Read the model definition and answer for the solid it produces. Units are mm, in the model's axes. Face numbers are marked on the shaded views. A direction names the side the tool comes from. Round coordinates to 2 decimals unless told otherwise and drop trailing zeros. Order: outer loops, then holes, each group sorted by start corner. A loop starts at its lowest first (then second) coordinate and runs counter-clockwise, first axis right, second up. Notation, with made-up numbers: (63.25, 65) - (69.25, 65) arc R16 ccw to (69.25, 93) - close; hole circle Ø7 at (21.25, 5.25). An arc over 180 degrees is marked (long way). One line per question, with ' | ' between items. Start each with the question number.
1) The part is cut by section A-A, the plane z = -6. Give the vertices of the cut face in (x, y), plus the area to 3 significant figures.
2) The mould has two halves that part along X. Classify the marked faces 6, 7, 8 and 9: pulls with the +X half, pulls with the -X half, needs draft (parallel to the pull), parting line crosses it, or undercut.
3) The part is cut by section B-B, the plane x = 31.1. Give the vertices of the cut face in (y, z).
4) The part is cut by section D-D, the plane y = -16.25. Give the vertices of the cut face in (x, z).
5) For the marked faces 1, 2, 3, 4 and 5, determine the directions among +Z, -Z, +X, -X, +Y, -Y from which every point of the face is accessible in a straight line to the end or side of a thin tool.
6) The part is cut by section C-C, the plane z = -10.5. Give the vertices of the cut face in (x, y).
7) Flat-ended cylindrical pins translate along their axes: pin 1 (3 mm diameter, centred on x = 31.1, y = -8.65, fed in from -Z); pin 2 (5 mm diameter, centred on x = 21, z = -32.5, fed in from +Y); pin 3 (4 mm diameter, centred on x = 31.5, z = -9, fed in from -Y); pin 4 (2.5 mm diameter, centred on x = 9.1, y = -8.65, fed in from -Z). Find the tip coordinate at first contact, or state that the pin passes through.
8) Straight lines are drawn through the part: line 1 (Z direction, x = 2, y = -14.25); line 2 (Z direction, x = 16, y = -10); line 3 (X direction, y = -3.35, z = -36.05). For each, find the intervals that lie inside material, in ascending order. Write a range as from..to.
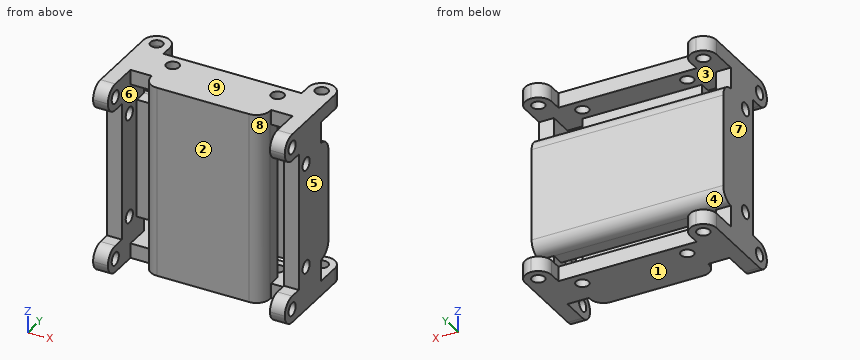
from build123d import *

# Parameters (mm, degrees)
ESBO_O1_R                  = 1.35
RESSALTO_EXTRUS_O1_DEPTH   = 2
ESBO_O3_W                  = 40.2
ESBO_O3_H                  = 2
RESSALTO_EXTRUS_O2_DEPTH   = 10.08
ESBO_O4_W                  = 3.1
ESBO_O4_H                  = 12.84
RESSALTO_EXTRUS_O3_DEPTH   = 34
CORTE_EXTRUS_O1_DEPTH      = 55.735280213
CORTE_EXTRUS_O1_DEPTH_BACK = 55.735280213
ESBO_O5_R                  = 1.35
ESBO_O7_W                  = 37.1
ESBO_O7_H                  = 3.24
CORTE_EXTRUS_O2_DEPTH      = 2
RESSALTO_EXTRUS_O5_START   = 2
ESBO_O12_R                 = 1.35
RESSALTO_EXTRUS_O5_DEPTH   = 2
ESBO_O18_W                 = 3.1
ESBO_O18_H                 = 3.24
RESSALTO_EXTRUS_O6_DEPTH   = 2
ESBO_O19_W                 = 3.1
ESBO_O19_H                 = 3.24
RESSALTO_EXTRUS_O7_DEPTH   = 2
ESBO_O21_R                 = 1.301764144
ESBO_O21_R_2               = 1.35
RESSALTO_EXTRUS_O8_DEPTH   = 1.1
RESSALTO_EXTRUS_O9_START   = 1.1
ESBO_O22_R                 = 1.35
RESSALTO_EXTRUS_O9_DEPTH   = 1.1
ESBO_O23_W                 = 3.1
ESBO_O23_H                 = 5.6
RESSALTO_EXTRUS_O10_DEPTH  = 5.85
CORTE_EXTRUS_O3_REACH      = 63.173
ESBO_O24_R                 = 1.35
ESBO_O25_W                 = 4.5
ESBO_O25_H                 = 3.1
CORTE_EXTRUS_O6_DEPTH      = 4.48
ESBO_O27_W                 = 3.1
ESBO_O27_H                 = 29
CORTE_EXTRUS_O7_DEPTH      = 4.48
ESBO_O28_W                 = 25
ESBO_O28_H                 = 40.2
CORTE_EXTRUS_O8_DEPTH      = 1.24
ESBO_O29_W                 = 25
ESBO_O29_H                 = 5.6
RESSALTO_EXTRUS_O11_DEPTH  = 34
ESBO_O31_W                 = 3.1
ESBO_O31_H                 = 25
RESSALTO_EXTRUS_O12_DEPTH  = 2.84
ESBO_O32_W                 = 25
ESBO_O32_H                 = 5.6
RESSALTO_EXTRUS_O13_DEPTH  = 34
FILETE1_R                  = 2.84
ESBO_O33_W                 = 5.6
ESBO_O33_H                 = 3.1
CORTE_EXTRUS_O9_DEPTH      = 0.55
ESBO_O35_W                 = 3.1
ESBO_O35_H                 = 5.6
CORTE_EXTRUS_O10_DEPTH     = 5.03
FILETE2_R                  = 2.8


with BuildPart() as part:
    # Esboço1 → Ressalto-extrusão1 (new body)
    with BuildSketch(Plane.XY):
        Polygon((0, 0), (5.6, 0), (5.6, -5.85), (34.6, -5.85), (34.6, 0), (40.2, 0), (40.2, -11.45), (0, -11.45), align=None)
        with Locations((2.8, -3.35)):
            Circle(ESBO_O1_R, mode=Mode.SUBTRACT)
        with Locations((37.4, -3.35)):
            Circle(ESBO_O1_R, mode=Mode.SUBTRACT)
        with Locations((31.1, -8.65)):
            Circle(ESBO_O1_R, mode=Mode.SUBTRACT)
        with Locations((9.1, -8.65)):
            Circle(ESBO_O1_R, mode=Mode.SUBTRACT)
    extrude(amount=RESSALTO_EXTRUS_O1_DEPTH)

    # Esboço3 → Ressalto-extrusão2 (add)
    with BuildSketch(Plane.XZ.offset(11.45)):
        with Locations((20.1, 1)):
            Rectangle(ESBO_O3_W, ESBO_O3_H)
    extrude(amount=RESSALTO_EXTRUS_O2_DEPTH)

    # Esboço4 → Ressalto-extrusão3 (add)
    with BuildSketch(Plane(origin=(0, 0, 0), x_dir=(-1, 0, 0), z_dir=(0, 0, -1))):
        with Locations((-38.65, -15.11)):
            Rectangle(ESBO_O4_W, ESBO_O4_H)
        with Locations((-1.55, -15.11)):
            Rectangle(ESBO_O4_W, ESBO_O4_H)
    extrude(amount=RESSALTO_EXTRUS_O3_DEPTH)

    # Esboço5 → Corte-extrusão1 (cut, two sides: drawn at the far end of the back side and taken through both)
    with BuildSketch(Plane.ZY.offset(-37.1).offset(-CORTE_EXTRUS_O1_DEPTH_BACK)):
        with Locations((-6, -14.25)):
            Circle(ESBO_O5_R)
        with Locations((-28, -14.25)):
            Circle(ESBO_O5_R)
    extrude(amount=CORTE_EXTRUS_O1_DEPTH + CORTE_EXTRUS_O1_DEPTH_BACK, mode=Mode.SUBTRACT)

    # Esboço7 → Corte-extrusão2 (cut)
    with BuildSketch(Plane(origin=(0, 0, 0), x_dir=(-1, 0, 0), z_dir=(0, 0, -1))):
        with Locations((-18.55, -19.91)):
            Rectangle(ESBO_O7_W, ESBO_O7_H)
    extrude(amount=-CORTE_EXTRUS_O2_DEPTH, mode=Mode.SUBTRACT)

    # Esboço12 → Ressalto-extrusão5 (add)
    with BuildSketch(Plane(origin=(0, 0, -34), x_dir=(-1, 0, 0), z_dir=(0, 0, -1)).offset(RESSALTO_EXTRUS_O5_START)):
        Polygon((-5.6, 0), (0, 0), (0, -18.29), (-40.2, -18.29), (-40.2, 0), (-34.6, 0), (-34.6, -5.85), (-5.6, -5.85), align=None)
        with Locations(Location((-31.1, -8.65, 0), (0, 0, 180))):
            Circle(ESBO_O12_R, mode=Mode.SUBTRACT)
        with Locations(Location((-9.1, -8.65, 0), (0, 0, 180))):
            Circle(ESBO_O12_R, mode=Mode.SUBTRACT)
        with Locations(Location((-2.8, -3.35, 0), (0, 0, 180))):
            Circle(ESBO_O12_R, mode=Mode.SUBTRACT)
        with Locations(Location((-37.4, -3.35, 0), (0, 0, 180))):
            Circle(ESBO_O12_R, mode=Mode.SUBTRACT)
    extrude(amount=-RESSALTO_EXTRUS_O5_DEPTH)

    # Esboço18 → Ressalto-extrusão6 (add)
    with BuildSketch(Plane.XY):
        with Locations((1.55, -19.91)):
            Rectangle(ESBO_O18_W, ESBO_O18_H)
    extrude(amount=RESSALTO_EXTRUS_O6_DEPTH)

    # Esboço19 → Ressalto-extrusão7 (add)
    with BuildSketch(Plane(origin=(0, 0, -34), x_dir=(-1, 0, 0), z_dir=(0, 0, -1))):
        with Locations((-1.55, -19.91)):
            Rectangle(ESBO_O19_W, ESBO_O19_H)
        with Locations((-38.65, -19.91)):
            Rectangle(ESBO_O19_W, ESBO_O19_H)
    extrude(amount=RESSALTO_EXTRUS_O7_DEPTH)

    # Esboço21 → Ressalto-extrusão8 (add)
    with BuildSketch(Plane.XY.offset(2)):
        Polygon((37.1, -21.53), (40.2, -21.53), (40.2, 0), (34.6, 0), (34.6, -5.85), (5.6, -5.85), (5.6, 0), (0, 0), (0, -21.53), (3.1, -21.53), (3.1, -18.29), (37.1, -18.29), align=None)
        with Locations((2.8, -3.35)):
            Circle(ESBO_O21_R, mode=Mode.SUBTRACT)
        with Locations((9.1, -8.65)):
            Circle(ESBO_O21_R_2, mode=Mode.SUBTRACT)
        with Locations((31.1, -8.65)):
            Circle(ESBO_O21_R_2, mode=Mode.SUBTRACT)
        with Locations((37.4, -3.35)):
            Circle(ESBO_O21_R_2, mode=Mode.SUBTRACT)
    extrude(amount=RESSALTO_EXTRUS_O8_DEPTH)

    # Esboço22 → Ressalto-extrusão9 (add)
    with BuildSketch(Plane(origin=(0, 0, -36), x_dir=(-1, 0, 0), z_dir=(0, 0, -1)).offset(RESSALTO_EXTRUS_O9_START)):
        Polygon((-5.6, 0), (0, 0), (0, -21.53), (-3.1, -21.53), (-3.1, -18.29), (-37.1, -18.29), (-37.1, -21.53), (-40.2, -21.53), (-40.2, 0), (-34.6, 0), (-34.6, -5.85), (-5.6, -5.85), align=None)
        with Locations(Location((-37.4, -3.35, 0), (0, 0, 180))):
            Circle(ESBO_O22_R, mode=Mode.SUBTRACT)
        with Locations(Location((-31.1, -8.65, 0), (0, 0, 180))):
            Circle(ESBO_O22_R, mode=Mode.SUBTRACT)
        with Locations(Location((-9.1, -8.65, 0), (0, 0, 180))):
            Circle(ESBO_O22_R, mode=Mode.SUBTRACT)
        with Locations(Location((-2.8, -3.35, 0), (0, 0, 180))):
            Circle(ESBO_O22_R, mode=Mode.SUBTRACT)
    extrude(amount=-RESSALTO_EXTRUS_O9_DEPTH)

    # Esboço23 → Ressalto-extrusão10 (add)
    with BuildSketch(Plane.XZ.offset(21.53)):
        with Locations((1.55, 0.3)):
            Rectangle(ESBO_O23_W, ESBO_O23_H)
        with Locations((1.55, -34.3)):
            Rectangle(ESBO_O23_W, ESBO_O23_H)
        with Locations((38.65, -34.3)):
            Rectangle(ESBO_O23_W, ESBO_O23_H)
        with Locations((38.65, 0.3)):
            Rectangle(ESBO_O23_W, ESBO_O23_H)
    extrude(amount=RESSALTO_EXTRUS_O10_DEPTH)

    # Corte-extrusão3: up to this face of the body (flat: up to its plane)
    corte_extrus_o3_end = Plane(part.part.faces().sort_by_distance((40.2, -15.177512698, -17))[0])
    # Esboço24 → Corte-extrusão3 (cut, up to the picked face)
    with BuildSketch(Plane.ZY, mode=Mode.PRIVATE) as corte_extrus_o3_sk1:
        with Locations(Location((-34.3, -19.55, 0), (0, 0, 270))):
            Circle(ESBO_O24_R)
    corte_extrus_o3_tool1 = split(extrude(corte_extrus_o3_sk1.sketch, amount=-CORTE_EXTRUS_O3_REACH, mode=Mode.PRIVATE), bisect_by=corte_extrus_o3_end, keep=Keep.BOTH, mode=Mode.PRIVATE)
    # Esboço24 → Corte-extrusão3 (cut, up to the picked face)
    with BuildSketch(Plane.ZY, mode=Mode.PRIVATE) as corte_extrus_o3_sk2:
        with Locations(Location((0.3, -19.55, 0), (0, 0, 270))):
            Circle(ESBO_O24_R)
    corte_extrus_o3_tool2 = split(extrude(corte_extrus_o3_sk2.sketch, amount=-CORTE_EXTRUS_O3_REACH, mode=Mode.PRIVATE), bisect_by=corte_extrus_o3_end, keep=Keep.BOTH, mode=Mode.PRIVATE)
    add(corte_extrus_o3_tool1.solids().sort_by(Axis((0, -19.55, -34.3), (1, 0, 0)))[0], mode=Mode.SUBTRACT)
    add(corte_extrus_o3_tool2.solids().sort_by(Axis((0, -19.55, 0.3), (1, 0, 0)))[0], mode=Mode.SUBTRACT)

    # Esboço25 → Corte-extrusão6 (cut)
    with BuildSketch(Plane.XZ.offset(18.29)):
        with Locations((5.35, -35.55)):
            Rectangle(ESBO_O25_W, ESBO_O25_H)
        with Locations((34.85, -35.55)):
            Rectangle(ESBO_O25_W, ESBO_O25_H)
        with Locations((34.85, 1.55)):
            Rectangle(ESBO_O25_W, ESBO_O25_H)
        with Locations((5.35, 1.55)):
            Rectangle(ESBO_O25_W, ESBO_O25_H)
    extrude(amount=-CORTE_EXTRUS_O6_DEPTH, mode=Mode.SUBTRACT)

    # Esboço27 → Corte-extrusão7 (cut)
    with BuildSketch(Plane.XZ.offset(21.53)):
        with Locations((1.55, -17)):
            Rectangle(ESBO_O27_W, ESBO_O27_H)
        with Locations((38.65, -17)):
            Rectangle(ESBO_O27_W, ESBO_O27_H)
    extrude(amount=-CORTE_EXTRUS_O7_DEPTH, mode=Mode.SUBTRACT)

    # Esboço28 → Corte-extrusão8 (cut)
    with BuildSketch(Plane.XZ.offset(18.29)):
        with Locations((20.1, -17)):
            Rectangle(ESBO_O28_W, ESBO_O28_H)
    extrude(amount=-CORTE_EXTRUS_O8_DEPTH, mode=Mode.SUBTRACT)

    # Esboço29 → Ressalto-extrusão11 (add)
    with BuildSketch(Plane.XY.offset(-34)):
        with Locations((20.1, -14.25)):
            Rectangle(ESBO_O29_W, ESBO_O29_H)
    extrude(amount=RESSALTO_EXTRUS_O11_DEPTH)

    # Esboço31 → Ressalto-extrusão12 (add)
    with BuildSketch(Plane(origin=(0, -8.69, 0), x_dir=(1, 0, 0), z_dir=(0, 1, 0))):
        with Locations((1.55, 17)):
            Rectangle(ESBO_O31_W, ESBO_O31_H)
        with Locations((38.65, 17)):
            Rectangle(ESBO_O31_W, ESBO_O31_H)
    extrude(amount=RESSALTO_EXTRUS_O12_DEPTH)

    # Esboço32 → Ressalto-extrusão13 (add)
    with BuildSketch(Plane.ZY.offset(-37.1)):
        with Locations((-17, -8.65)):
            Rectangle(ESBO_O32_W, ESBO_O32_H)
    extrude(amount=RESSALTO_EXTRUS_O13_DEPTH)

    # Filete1
    filete1_edges = [part.edges().sort_by_distance(p)[0] for p in [
        (32.6, -17.05, -17),
        (7.6, -17.05, -17),
        (20.1, -5.85, -29.5),
        (20.1, -5.85, -4.5),
    ]]
    fillet(filete1_edges, radius=FILETE1_R)

    # Esboço33 → Corte-extrusão9 (cut)
    with BuildSketch(Plane(origin=(0, 0, 0), x_dir=(1, 0, 0), z_dir=(0, 1, 0))):
        with Locations((2.8, 35.55)):
            Rectangle(ESBO_O33_W, ESBO_O33_H)
        with Locations((37.4, 35.55)):
            Rectangle(ESBO_O33_W, ESBO_O33_H)
        with Locations((37.4, -1.55)):
            Rectangle(ESBO_O33_W, ESBO_O33_H)
        with Locations((2.8, -1.55)):
            Rectangle(ESBO_O33_W, ESBO_O33_H)
    extrude(amount=-CORTE_EXTRUS_O9_DEPTH, mode=Mode.SUBTRACT)

    # Esboço35 → Corte-extrusão10 (cut)
    with BuildSketch(Plane.XZ.offset(27.38)):
        with Locations((1.55, 0.3)):
            Rectangle(ESBO_O35_W, ESBO_O35_H)
        with Locations((38.65, 0.3)):
            Rectangle(ESBO_O35_W, ESBO_O35_H)
        with Locations((38.65, -34.3)):
            Rectangle(ESBO_O35_W, ESBO_O35_H)
        with Locations((1.55, -34.3)):
            Rectangle(ESBO_O35_W, ESBO_O35_H)
    extrude(amount=-CORTE_EXTRUS_O10_DEPTH, mode=Mode.SUBTRACT)

    # Filete2
    filete2_edges = [part.edges().sort_by_distance(p)[0] for p in [
        (34.6, -0.55, 1.55),
        (40.2, -0.55, 1.55),
        (0, -0.55, 1.55),
        (5.6, -0.55, 1.55),
        (40.2, -0.55, -35.55),
        (34.6, -0.55, -35.55),
        (5.6, -0.55, -35.55),
        (0, -0.55, -35.55),
        (1.55, -22.35, -31.5),
        (1.55, -22.35, -37.1),
        (38.65, -22.35, -37.1),
        (38.65, -22.35, -31.5),
        (38.65, -22.35, -2.5),
        (38.65, -22.35, 3.1),
        (1.55, -22.35, -2.5),
        (1.55, -22.35, 3.1),
    ]]
    fillet(filete2_edges, radius=FILETE2_R - 0.0001)  # a hair under: the kernel refuses the full size


solid = part.part
Values:
1) outline: (0, -17.05) - (3.1, -17.05) - (3.1, -15.6) - (0, -15.6) - close; (0, -12.9) - (3.1, -12.9) - (3.1, -11.45) - (7.6, -11.45) - (7.6, -14.21) arc R2.84 ccw to (10.44, -17.05) - (29.76, -17.05) arc R2.84 ccw to (32.6, -14.21) - (32.6, -11.45) - (37.1, -11.45) - (37.1, -12.9) - (40.2, -12.9) - (40.2, -6.19) - (0, -6.19) - close; (37.1, -17.05) - (40.2, -17.05) - (40.2, -15.6) - (37.1, -15.6) - close | area: 366 mm^2
2) face 6: undercut | face 7: pulls with the -X half | face 8: undercut | face 9: needs draft
3) outline: (-16.71, -37.1) - (-10, -37.1) - (-10, -34) - (-11.45, -34) - (-11.45, -29.5) - (-8.69, -29.5) arc R2.84 ccw to (-5.85, -26.66) - (-5.85, -7.34) arc R2.84 ccw to (-8.69, -4.5) - (-11.45, -4.5) - (-11.45, 0) - (-10, 0) - (-10, 3.1) - (-16.71, 3.1) - close; (-7.3, -37.1) - (-5.85, -37.1) - (-5.85, -34) - (-7.3, -34) - close; (-7.3, 0) - (-5.85, 0) - (-5.85, 3.1) - (-7.3, 3.1) - close
4) outline: (0, -37.1) - (3.1, -37.1) - (3.1, 3.1) - (0, 3.1) - close; (8.46, -37.1) - (31.74, -37.1) - (31.74, 3.1) - (8.46, 3.1) - close; (37.1, -37.1) - (40.2, -37.1) - (40.2, 3.1) - (37.1, 3.1) - close
5) face 1: -Z, +X, -X, +Y, -Y | face 2: +Z, -Z, -Y | face 3: +Y | face 4: +X, -X, +Y | face 5: +Z, -Z, +X, +Y, -Y
6) outline: (0, -17.05) - (3.1, -17.05) - (3.1, -11.45) - (7.6, -11.45) - (7.6, -14.21) arc R2.84 ccw to (10.44, -17.05) - (29.76, -17.05) arc R2.84 ccw to (32.6, -14.21) - (32.6, -11.45) - (37.1, -11.45) - (37.1, -17.05) - (40.2, -17.05) - (40.2, -5.85) - (0, -5.85) - close
7) pin 1: stops at z = -37.1 | pin 2: stops at y = -5.85 | pin 3: stops at y = -17.05 | pin 4: stops at z = -29.5
8) line 1: z = -37.1..-29.35, -26.65..-7.35, -4.65..3.1 | line 2: z = -37.1..-34, -29.5..-4.5, 0..3.1 | line 3: x = 0..1.45, 4.15..5.6, 34.6..36.05, 38.75..40.2
